Autodesk Inventor part; units mm, degrees
ref_plane "YZ Plane" through (0, 0, 0) normal (1, 0, 0) x (0, 1, 0)
ref_plane "XZ Plane" through (0, 0, 0) normal (0, 1, 0) x (-1, 0, 0)
ref_plane "XY Plane" through (0, 0, 0) normal (0, 0, 1) x (1, 0, 0)
sketch "Sketch2" plane through (0, 0, 0) normal (0, 1, 0) x (-1, 0, 0)
  line L0 (-17, 32.5) -> (17, 32.5)
  line L1 (17, 32.5) -> (17, -32.5)
  line L2 (17, -32.5) -> (-17, -32.5)
  line L3 (-17, -32.5) -> (-17, 32.5)
  line L4 (-17, 32.5) -> (17, -32.5) construction
  line L5 (17, 32.5) -> (-17, -32.5) construction
  line L6 (0, 30.5) -> (-15, 30.5)
  line L7 (-15, 30.5) -> (-15, 17.5)
  line L8 (-15, 17.5) -> (0, 17.5)
  line L9 (0, 17.5) -> (0, 30.5)
  line L10 (0, 15.5) -> (15, 15.5)
  line L11 (15, 15.5) -> (15, 2.5)
  line L12 (15, 2.5) -> (0, 2.5)
  line L13 (0, 2.5) -> (0, 15.5)
  line L14 (-7.5, 0.5) -> (-15, 0.5)
  line L15 (-15, 0.5) -> (-15, -12.5)
  line L16 (-15, -12.5) -> (-7.5, -12.5)
  line L17 (-7.5, -12.5) -> (-7.5, 0.5)
  line L18 (15, -14.5) -> (7.5, -14.5)
  line L19 (7.5, -14.5) -> (7.5, -27.5)
  line L20 (7.5, -27.5) -> (15, -27.5)
  line L21 (15, -27.5) -> (15, -14.5)
  point P0 (0, 0)
  dimension "d35" = 34
  dimension "d36" = 65
  dimension "d37" = 15
  dimension "d38" = 13
  dimension "d39" = 15
  dimension "d40" = 13
  dimension "d41" = 2
  dimension "d42" = 2
  dimension "d43" = 0
  dimension "d44" = 2
  dimension "d45" = 7.5
  dimension "d46" = 13
  dimension "d47" = 7.5
  dimension "d48" = 2
  dimension "d49" = 7.5
  dimension "d50" = 13
  dimension "d51" = 2
  dimension "d52" = 2
extrude "Extrusion4" add sketch "Sketch2" along normal blind 2
sketch "Sketch3" plane through (0, 0, 0) normal (0, 1, 0) x (-1, 0, 0)
  circle A0 centre (0, 57.5) radius 97.6 construction
  line L0 (17, 32.5) -> (-17, 32.5)
  point P0 (0, 0)
  dimension "d55" = 195.2
  dimension "d56" = 25
properties part number "Molecule Chopper"
Source: CAD feature listing. Evaluate the final solid. Frame: model axes, mm. A direction names the side the tool comes from. Coordinates: 2 decimals unless noted, no trailing zeros. Write each loop counter-clockwise with the first axis right and the second up, starting at its lowest first coordinate (ties: lowest second). Pieces come first, ordered by that corner, then holes. Notation, with made-up numbers: M 63.25,29.25 L 122.25,29.25 A8 ccw 122.25,38.25 Z; hole C -31,-9.5 d1. An arc over 180 degrees is marked long. Use a Markdown table: item, result.
1) Section B-B, the plane x = 6.5. Output: boundary loops of the cut face in (y, z).
Conclusion:
| item | result |
|---|---|
| outline | M 0,-32.5 L 2,-32.5 L 2,17.5 L 0,17.5 Z; M 0,30.5 L 2,30.5 L 2,32.5 L 0,32.5 Z |
2) Mould query, pull axis X, two halves, no side actions, for faces 1 (the flat face through (-11, 1, -27.5)), 2 (the flat face through (-17, 1, 0)), 3 (the flat face through (0, 0, -7)), 4 (the flat face through (0, 1, 9)). Classes: pulls with the +X half, pulls with the -X half, needs draft (parallel to the pull), parting line crosses it, or undercut.
Conclusion:
| item | result |
|---|---|
| face 1 | undercut |
| face 2 | pulls with the -X half |
| face 3 | needs draft |
| face 4 | undercut |
3) Section D-D, the plane y = 1.45. Output: boundary loops of the cut face in (x, z).
Conclusion:
| item | result |
|---|---|
| outline | M -17,-32.5 L 17,-32.5 L 17,32.5 L -17,32.5 Z; hole M -15,-27.5 L -7.5,-27.5 L -7.5,-14.5 L -15,-14.5 Z; hole M -15,2.5 L 0,2.5 L 0,15.5 L -15,15.5 Z; hole M 0,17.5 L 15,17.5 L 15,30.5 L 0,30.5 Z; hole M 7.5,-12.5 L 15,-12.5 L 15,0.5 L 7.5,0.5 Z |
4) Section A-A, the plane z = -5.5. Output: boundary loops of the cut face in (x, y), then the cut area to 3 significant figures.
Conclusion:
| item | result |
|---|---|
| outline | M -17,0 L 7.5,0 L 7.5,2 L -17,2 Z; M 15,0 L 17,0 L 17,2 L 15,2 Z |
| area | 53.0 mm^2 |
5) Ray query, L1, parallel to Z at x = 13.5, y = 0.2; L2, parallel to X at y = 1.8, z = 20.5; L3, parallel to Z at x = 2, y = 1.75. Return the intervals inside material, ascending.
Conclusion:
| item | result |
|---|---|
| L1 | z = -32.5 to -12.5, 0.5 to 17.5, 30.5 to 32.5 |
| L2 | x = -17 to 0, 15 to 17 |
| L3 | z = -32.5 to 17.5, 30.5 to 32.5 |
6) Section C-C, the plane x = -11. Output: boundary loops of the cut face in (y, z).
Conclusion:
| item | result |
|---|---|
| outline | M 0,-32.5 L 2,-32.5 L 2,-27.5 L 0,-27.5 Z; M 0,-14.5 L 2,-14.5 L 2,2.5 L 0,2.5 Z; M 0,15.5 L 2,15.5 L 2,32.5 L 0,32.5 Z |
7) Reachability of faces 5 (the flat face through (0, 1, -32.5)), 6 (the flat face through (11, 1, -12.5)) from +Z, -Z, +X, -X, +Y, -Y: full face, straight path, thin tool, end or side. Return the list, or none.
Conclusion:
| item | result |
|---|---|
| face 5 | -Z, +X, -X, +Y, -Y |
| face 6 | +Y, -Y |
